```python
from build123d import *

# Parameters (mm, degrees)
BOSS_EXTRUDE1_DEPTH = 10
FILLET1_R           = 1
FILLET2_R           = 5


with BuildPart() as part:
    # Sketch1 → Boss-Extrude1 (new body)
    with BuildSketch(Plane(origin=(0, 0, 0), x_dir=(1, 0, 0), z_dir=(0, 1, 0))):
        with BuildLine():
            Line((-5.303300859, 15.303300859), (-7.424621202, 17.424621202))
            ThreePointArc((-7.424621202, 17.424621202), (-10.438158184, 8.862083601), (-5.650442461, 1.15))
            ThreePointArc((-5.650442461, 1.15), (-12.343952667, -8.031032616), (-8.838834765, -18.838834765))
            Line((-8.838834765, -18.838834765), (-6.717514421, -16.717514421))
            ThreePointArc((-6.717514421, -16.717514421), (0, -0.5), (6.717514421, -16.717514421))
            Line((6.717514421, -16.717514421), (8.838834765, -18.838834765))
            ThreePointArc((8.838834765, -18.838834765), (12.343952667, -8.031032616), (5.650442461, 1.15))
            ThreePointArc((5.650442461, 1.15), (10.438158184, 8.862083601), (7.424621202, 17.424621202))
            Line((7.424621202, 17.424621202), (5.303300859, 15.303300859))
            ThreePointArc((5.303300859, 15.303300859), (0, 2.5), (-5.303300859, 15.303300859))
        make_face()
    extrude(amount=BOSS_EXTRUDE1_DEPTH)

    # Fillet1
    fillet1_edges = [part.edges().sort_by_distance(p)[0] for p in [
        (5.303300859, 5, -15.303300859),
        (7.424621202, 5, -17.424621202),
        (8.838834765, 5, 18.838834765),
        (6.717514421, 5, 16.717514421),
        (-6.717514421, 5, 16.717514421),
        (-8.838834765, 5, 18.838834765),
        (-7.424621202, 5, -17.424621202),
        (-5.303300859, 5, -15.303300859),
    ]]
    fillet(fillet1_edges, radius=FILLET1_R)

    # Fillet2
    fillet2_edges = [part.edges().sort_by_distance(p)[0] for p in [
        (5.650442461, 5, -1.15),
        (-5.650442461, 5, -1.15),
    ]]
    fillet(fillet2_edges, radius=FILLET2_R)


solid = part.part
```
CAD build for the part. Positions are in the model's coordinates, mm. A direction names the side the tool comes from. Give positions to 0.01 mm unless a question says otherwise; leave off trailing zeros. Order: outer loops, then holes, each group sorted by start corner. A loop starts at its lowest first (then second) coordinate and runs counter-clockwise, first axis right, second up. Notation, with made-up numbers: M 72.25,82 L 87.25,82 A20 cw 87.25,93 Z; hole C 79,54.5 d6. An arc over 180 degrees is marked long. Put each result on its own line as item: value. Start each with the question number.
(1) Saw through at C-C, the plane z = 14.5. Write the cut outline in (x, y).
(2) Which spindle directions (+Z, -Z, +X, -X, +Y, -Y) get a long thin tool onto all of the face, cutting with end or side? Do faces 4 (the flat face through (1, 0, -1)), 5 (the cylindrical face through (7.1, 5.1, 16.7)). Say none if no direction does.
(3) Mould opens along Z. For faces 1 (the cylindrical face through (-7.428, 5.07, -16.972)), 2 (the flat face through (1, 10, -1)), 3 (the cylindrical face through (-0.301, 4.93, 0.505)) say: +Z half, -Z half, draft (parallel to the pull), parting line (faces both ways), or undercut.
(4) Flat gauge pins, fed straight in: pin 1 Ø12 at (x, z) = (7, 4) entering from -Y; pin 2 Ø1 at (x, y) = (0, 7) entering from -Z; pin 3 Ø1.5 at (x, z) = (8, 10) entering from +Y; pin 4 Ø1 at (x, y) = (8, 5) entering from +Z. Where does each tip first touch, or does it go through?
(5) Saw through at D-D, the plane x = 3. Write the cut outline in (y, z), then the cut area to 3 significant figures.
(6) Drill centre lines: line 1 along X through (y, z) = (4.5, -10); line 2 along X through (y, z) = (4.25, 10); line 3 along Z through (x, y) = (0, 6). Where is each one in solid material? Low to high.
(7) Saw through at A-A, the plane z = 10. Write the cut outline in (x, y), then the cut area to 3 significant figures.
(8) Saw through at B-B, the plane x = 0. Write the cut outline in (y, z).
Check result:
1. outline: M -11.66,0 L -8.37,0 L -8.37,10 L -11.66,10 Z; M 8.37,0 L 11.66,0 L 11.66,10 L 8.37,10 Z
2. face 4: +Z, -Z, +X, -X, -Y
2. face 5: +Y, -Y
3. face 1: -Z half
3. face 2: draft
3. face 3: undercut
4. pin 1: stops at y = 0
4. pin 2: stops at z = -2.52
4. pin 3: passes through
4. pin 4: stops at z = 18.35
5. outline: M 0,-3.13 L 10,-3.13 L 10,0.99 L 0,0.99 Z
5. area: 41.1 mm2
6. line 1: x = -10.5 to -7.5, 7.5 to 10.5
6. line 2: x = -12.5 to -9.5, 9.5 to 12.5
6. line 3: z = -2.5 to 0.5
7. outline: M -12.5,0 L -9.5,0 L -9.5,10 L -12.5,10 Z; M 9.5,0 L 12.5,0 L 12.5,10 L 9.5,10 Z
7. area: 60.0 mm2
8. outline: M 0,-2.5 L 10,-2.5 L 10,0.5 L 0,0.5 Z
